```python
from build123d import *

# Parameters (mm, degrees)
SKETCH1_W                        = 300
SKETCH1_H                        = 150
PCB_BASE_DEPTH                   = 1
SKETCH2_R                        = 10
SKETCH2_R_2                      = 15
SKETCH2_RX                       = 35
SKETCH2_RY                       = 15
SKETCH2_W                        = 35
SKETCH2_H                        = 25
SKETCH2_H_2                      = 32
PCB_CHIPS_DEPTH                  = 4
SLOT_CUT_DEPTH                   = 10
F_10_0MM_DOWEL_HOLE1_D           = 10
F_10_0MM_DOWEL_HOLE1_DEPTH       = 10
F_10_0MM_DOWEL_HOLE1_CSINK_D     = 10.05
F_10_0MM_DOWEL_HOLE1_CSINK_ANGLE = 90
F_10_0MM_DOWEL_HOLE1_TIP         = 3.004303095
FILLET1_R                        = 10
CHAMFER1_SIZE                    = 10


with BuildPart() as part:
    # Sketch1 → PCB Base (new body, symmetric)
    with BuildSketch(Plane.XY):
        with Locations((-150, 75)):
            Rectangle(SKETCH1_W, SKETCH1_H)
    extrude(amount=PCB_BASE_DEPTH, both=True)

    # Sketch2 → PCB Chips (add)
    with BuildSketch(Plane.XY.offset(1)):
        with Locations((-260, 85)):
            Circle(SKETCH2_R)
        with Locations((-220, 85)):
            Circle(SKETCH2_R)
        with Locations((-240, 60)):
            Circle(SKETCH2_R_2)
        with Locations((-240, 60)):
            Circle(SKETCH2_R, mode=Mode.SUBTRACT)
        with Locations((-60, 60)):
            Circle(SKETCH2_R_2)
        with Locations((-60, 60)):
            Circle(SKETCH2_R, mode=Mode.SUBTRACT)
        with Locations((-80, 85)):
            Circle(SKETCH2_R)
        with Locations((-40, 85)):
            Circle(SKETCH2_R)
        with Locations((-240, 120)):
            Ellipse(SKETCH2_RX, SKETCH2_RY)
        with Locations((-60, 120)):
            Ellipse(SKETCH2_RX, SKETCH2_RY)
        with Locations((-177.5, 50.5)):
            Rectangle(SKETCH2_W, SKETCH2_H)
        with Locations((-177.5, 89)):
            Rectangle(SKETCH2_W, SKETCH2_H_2)
        Polygon((-195, 110), (-160, 110), (-160, 125), (-177.320508076, 135), (-195, 135), align=None)
        Polygon((-140, 125), (-122.679491924, 135), (-105, 135), (-105, 110), (-140, 110), align=None)
        with Locations((-122.5, 89)):
            Rectangle(SKETCH2_W, SKETCH2_H_2)
        with Locations((-122.5, 50.5)):
            Rectangle(SKETCH2_W, SKETCH2_H)
    pcb_chips = extrude(amount=PCB_CHIPS_DEPTH)

    # Mirror Chips: PCB Chips across plane
    add(pcb_chips.mirror(Plane.XY))

    # Sketch3 → Slot Cut (cut)
    with BuildSketch(Plane.XY.offset(1)):
        with BuildLine():
            Line((-272.5, 37.5), (-272.5, 0))
            Line((-272.5, 0), (-267.5, 0))
            Line((-267.5, 0), (-267.5, 37.5))
            ThreePointArc((-267.5, 37.5), (-270, 40), (-272.5, 37.5))
        make_face()
        with BuildLine():
            Line((-32.5, 0), (-32.5, 37.5))
            ThreePointArc((-32.5, 37.5), (-30, 40), (-27.5, 37.5))
            Line((-27.5, 37.5), (-27.5, 0))
            ThreePointArc((-27.5, 0), (-30, -2.5), (-32.5, 0))
        make_face()
    extrude(amount=-SLOT_CUT_DEPTH, mode=Mode.SUBTRACT)

    # Ø10.0mm Dowel Hole1
    with Locations(Plane.XY.offset(1)):
        with Locations((-285, 100), (-285, 20), (-15, 20), (-15, 100)):
            CounterSinkHole(F_10_0MM_DOWEL_HOLE1_D / 2, F_10_0MM_DOWEL_HOLE1_CSINK_D / 2, depth=F_10_0MM_DOWEL_HOLE1_DEPTH, counter_sink_angle=F_10_0MM_DOWEL_HOLE1_CSINK_ANGLE)
            with Locations((0, 0, -(F_10_0MM_DOWEL_HOLE1_DEPTH + F_10_0MM_DOWEL_HOLE1_TIP / 2))):  # 118° drill point
                Cone(0, F_10_0MM_DOWEL_HOLE1_D / 2, F_10_0MM_DOWEL_HOLE1_TIP, mode=Mode.SUBTRACT)

    # Fillet1
    fillet1_edges = [part.edges().sort_by_distance(p)[0] for p in [
        (0, 150, 0),
        (-300, 150, 0),
    ]]
    fillet(fillet1_edges, radius=FILLET1_R)

    # Chamfer1
    chamfer1_edges = [part.edges().sort_by_distance(p)[0] for p in [
        (0, 0, 0),
        (-300, 0, 0),
    ]]
    chamfer(chamfer1_edges, length=CHAMFER1_SIZE)


solid = part.part
```
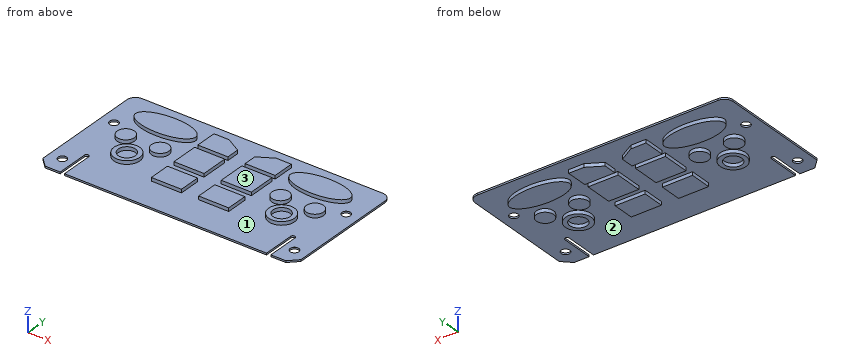
Here's how the part is built. I have some questions about the finished solid (model axes, mm). Face numbers are marked on the shaded views. Coordinates: 2 decimals unless noted, no trailing zeros. Order: outer loops, then holes, each group sorted by start corner. A loop starts at its lowest first (then second) coordinate and runs counter-clockwise, first axis right, second up. Notation, with made-up numbers: M 50.25,40.25 L 61.25,40.25 A37 ccw 61.25,77.25 Z; hole C 52,22.5 d2. An arc over 180 degrees is marked long. Answer as a JSON object with one key per item and string values. Group by question number.
(1) Suppose I cut it at D-D, the plane x = -192. Please give me the cut outline in (y, z).
(2) For pin 1 (3 mm diameter, centred on y = 45.5, z = -3, fed in from -X); pin 2 (23 mm diameter, centred on x = -240, y = 60, fed in from +Z); pin 3 (4.5 mm diameter, centred on y = 123, z = 3.5, fed in from +X); pin 4 (1 mm diameter, centred on y = 83.5, z = -2, fed in from +X), each with a flat end and sliding along its axis, tell me the tip position at first contact or that it passes through.
(3) If we mould it in two halves opening along X, with no side actions, what happens to the marked faces 1, 2 and 3? For each: released by +X, released by -X, zero draft, split by the parting line, or undercut.
(4) Suppose I cut it at A-A, the plane x = -285. Please give me the cut outline in (y, z) (3 decimals), then the cut area to 3 significant figures.
(5) Suppose I cut it at B-B, the plane y = 100. State how many separate pieces and enclosed holes the cut face has, then the cut area to 3 significant figures.
(6) I need wall thicknesses on probe 1 along X at (y, z) = (59, -4.25); probe 2 along Y at (x, z) = (-240, -3.5); probe 3 along Y at (x, z) = (-15, 0.4). Which ranges of each line are inside material? Lowest first, please.
Values found:
{
 "1": {"outline": "M 0,-1 L 38,-1 L 38,-5 L 63,-5 L 63,-1 L 73,-1 L 73,-5 L 105,-5 L 105,-1 L 110,-1 L 110,-5 L 135,-5 L 135,-1 L 150,-1 L 150,1 L 135,1 L 135,5 L 110,5 L 110,1 L 105,1 L 105,5 L 73,5 L 73,1 L 63,1 L 63,5 L 38,5 L 38,1 L 0,1 Z"},
 "2": {"pin 1": "stops at x = -247.48", "pin 2": "stops at z = 5", "pin 3": "stops at x = -25.04", "pin 4": "stops at x = -30.05"},
 "3": {"face 1": "undercut", "face 2": "undercut", "face 3": "zero draft"},
 "4": {"outline": "M 0,-1 L 15,-1 L 15,0.975 L 14.975,1 L 0,1 Z; M 25,-1 L 95,-1 L 95,0.975 L 94.975,1 L 25.025,1 L 25,0.975 Z; M 105,-1 L 150,-1 L 150,1 L 105.025,1 L 105,0.975 Z", "area": "260 mm^2"},
 "5": {"separate pieces": "3", "enclosed holes": "0", "area": "1,120 mm^2"},
 "6": {"probe 1": "x = -254.97 to -249.95, -230.05 to -225.03, -195 to -160, -140 to -105, -74.97 to -69.95, -50.05 to -45.03", "probe 2": "y = 45 to 50, 70 to 75, 105 to 135", "probe 3": "y = 0 to 15, 25 to 95, 105 to 150"}
}
